```python
from build123d import *

# Parameters (mm, degrees)
SKETCH1_R           = 1.6
BOSS_EXTRUDE1_DEPTH = 1.6
SKETCH3_W           = 15
SKETCH3_H           = 14
BOSS_EXTRUDE2_DEPTH = 3


with BuildPart() as part:
    # Sketch1 → Boss-Extrude1 (new body)
    with BuildSketch(Plane.XY):
        with BuildLine():
            Line((-13.235657624, 13.611622239), (16.764342376, 13.611622239))
            ThreePointArc((16.764342376, 13.611622239), (18.178555938, 13.025835801), (18.764342376, 11.611622239))
            Line((18.764342376, 11.611622239), (18.764342376, -18.388377761))
            ThreePointArc((18.764342376, -18.388377761), (18.178555938, -19.802591324), (16.764342376, -20.388377761))
            Line((16.764342376, -20.388377761), (-13.235657624, -20.388377761))
            ThreePointArc((-13.235657624, -20.388377761), (-14.649871187, -19.802591324), (-15.235657624, -18.388377761))
            Line((-15.235657624, -18.388377761), (-15.235657624, 11.611622239))
            ThreePointArc((-15.235657624, 11.611622239), (-14.649871187, 13.025835801), (-13.235657624, 13.611622239))
        make_face()
        with Locations((16.764342376, 11.611622239)):
            Circle(SKETCH1_R, mode=Mode.SUBTRACT)
        with Locations(Location((16.764342376, -18.388377761, 0), (0, 0, 180))):
            Circle(SKETCH1_R, mode=Mode.SUBTRACT)
        with Locations(Location((-13.235657624, 11.611622239, 0), (0, 0, 180))):
            Circle(SKETCH1_R, mode=Mode.SUBTRACT)
        with Locations((-13.235657624, -18.388377761)):
            Circle(SKETCH1_R, mode=Mode.SUBTRACT)
    extrude(amount=BOSS_EXTRUDE1_DEPTH)

    # Sketch3 → Boss-Extrude2 (add)
    with BuildSketch(Plane.XY.offset(1.6)):
        with Locations((1.764342376, 1.611622239)):
            Rectangle(SKETCH3_W, SKETCH3_H)
    extrude(amount=BOSS_EXTRUDE2_DEPTH)


solid = part.part
```
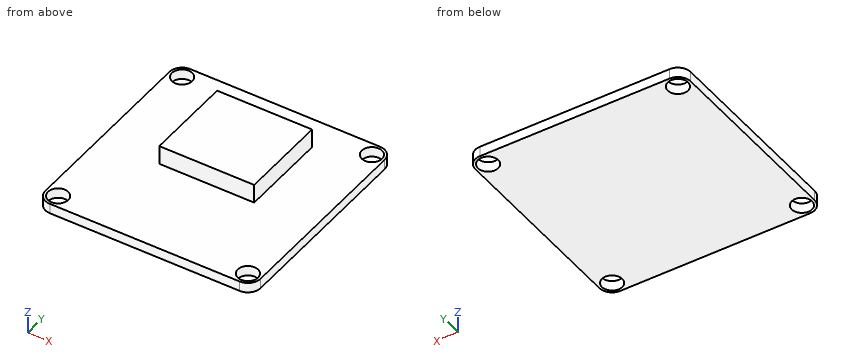
For this review, take the finished solid that the model builds, in its own axes (mm). Coordinates: 2 decimals unless noted, no trailing zeros. Order: outer loops, then holes, each group sorted by start corner. A loop starts at its lowest first (then second) coordinate and runs counter-clockwise, first axis right, second up. Notation, with made-up numbers: (-39.5, 4.5) -> (18.5, 4.5) arc R32 ccw to (18.5, 43.5) -> close; hole circle Ø9 at (72.5, 20). An arc over 180 degrees is marked (long way). Answer as CSV lines item,"result".
Q1. We need section C-C (y = 2). State the section outline as (x, z) points.
Model answer:
outline,"(-15.24, 0) -> (18.76, 0) -> (18.76, 1.6) -> (9.26, 1.6) -> (9.26, 4.6) -> (-5.74, 4.6) -> (-5.74, 1.6) -> (-15.24, 1.6) -> close"
Q2. We need section A-A (z = 0.75). State the section outline as (x, y) points.
Model answer:
outline,"(-15.24, -18.39) arc R2 ccw to (-13.24, -20.39) -> (16.76, -20.39) arc R2 ccw to (18.76, -18.39) -> (18.76, 11.61) arc R2 ccw to (16.76, 13.61) -> (-13.24, 13.61) arc R2 ccw to (-15.24, 11.61) -> close; hole circle Ø3.2 at (-13.24, -18.39); hole circle Ø3.2 at (-13.24, 11.61); hole circle Ø3.2 at (16.76, -18.39); hole circle Ø3.2 at (16.76, 11.61)"
Q3. We need section B-B (x = -12.5). State the section outline as (y, z) points.
Model answer:
outline,"(-20.39, 0) -> (-19.81, 0) -> (-19.81, 1.6) -> (-20.39, 1.6) -> close; (-16.97, 0) -> (10.19, 0) -> (10.19, 1.6) -> (-16.97, 1.6) -> close; (13.03, 0) -> (13.61, 0) -> (13.61, 1.6) -> (13.03, 1.6) -> close"
Q4. We need section D-D (x = 5). State the section outline as (y, z) points, plus the area to 3 significant figures.
Model answer:
outline,"(-20.39, 0) -> (13.61, 0) -> (13.61, 1.6) -> (8.61, 1.6) -> (8.61, 4.6) -> (-5.39, 4.6) -> (-5.39, 1.6) -> (-20.39, 1.6) -> close"
area,"96.4 mm2"
Q5. Wall thickness on line 1 along X through (y, z) = (-18, 0.55); line 2 along Z through (x, y) = (-13, -14.5); line 3 along Y through (x, z) = (0.5, 3.8): over which ranges is each line inside the solid? List them lowest first. Write a range as [from, to].
Model answer:
line 1,"x = [-15.24, -14.79], [-11.68, 15.21], [18.32, 18.76]"
line 2,"z = [0, 1.6]"
line 3,"y = [-5.39, 8.61]"
Q6. Clearance check with flat-ended pins moving along their axes: pin 1 Ø1 at (y, z) = (-1, 3) entering from +X; pin 2 Ø5 at (x, y) = (-13.24, 11.61) entering from +Z; pin 3 Ø0.9 at (x, z) = (0.5, 3) entering from +Y. State where each tip first meets the part, or that it passes through.
Model answer:
pin 1,"stops at x = 9.26"
pin 2,"stops at z = 1.6"
pin 3,"stops at y = 8.61"
